from build123d import *

# Parameters (mm, degrees)
CROQUIS3_W              = 38
CROQUIS3_H              = 21.5
SALIENTE_EXTRUIR2_DEPTH = 60
CROQUIS4_R              = 4.1
CORTAR_EXTRUIR2_DEPTH   = 60
CROQUIS5_W              = 20
CROQUIS5_H              = 2
CORTAR_EXTRUIR4_DEPTH   = 39
CROQUIS6_R              = 3.5
CORTAR_EXTRUIR5_DEPTH   = 3
CROQUIS7_R              = 1.55
CORTAR_EXTRUIR6_DEPTH   = 22
CROQUIS8_R              = 4.5
CORTAR_EXTRUIR7_DEPTH   = 3
CROQUIS9_R              = 1.5
CORTAR_EXTRUIR8_DEPTH   = 15
CROQUIS10_W             = 38
CROQUIS10_H             = 0.5
CORTAR_EXTRUIR9_DEPTH   = 60


with BuildPart() as part:
    # Croquis3 → Saliente-Extruir2 (new body)
    with BuildSketch(Plane(origin=(0, 0, 0), x_dir=(0, 0, -1), z_dir=(1, 0, 0))):
        Rectangle(CROQUIS3_W, CROQUIS3_H)
    extrude(amount=SALIENTE_EXTRUIR2_DEPTH)

    # Croquis4 → Cortar-Extruir2 (cut)
    with BuildSketch(Plane(origin=(60, 0, 0), x_dir=(0, 0, -1), z_dir=(1, 0, 0))):
        with Locations((-10, 0)):
            Circle(CROQUIS4_R)
        with Locations((10, 0)):
            Circle(CROQUIS4_R)
    extrude(amount=-CORTAR_EXTRUIR2_DEPTH, mode=Mode.SUBTRACT)

    # Croquis5 → Cortar-Extruir4 (cut)
    with BuildSketch(Plane.XY.offset(19)):
        with Locations((50, 0)):
            Rectangle(CROQUIS5_W, CROQUIS5_H)
    extrude(amount=-CORTAR_EXTRUIR4_DEPTH, mode=Mode.SUBTRACT)

    # Croquis6 → Cortar-Extruir5 (cut)
    with BuildSketch(Plane.XZ.offset(10.75)):
        with Locations(Location((54, 0, 0), (0, 0, 270))):
            Circle(CROQUIS6_R)
    extrude(amount=-CORTAR_EXTRUIR5_DEPTH, mode=Mode.SUBTRACT)

    # Croquis7 → Cortar-Extruir6 (cut)
    with BuildSketch(Plane.XZ.offset(10.75)):
        with Locations(Location((54, 0, 0), (0, 0, 270))):
            Circle(CROQUIS7_R)
    extrude(amount=-CORTAR_EXTRUIR6_DEPTH, mode=Mode.SUBTRACT)

    # Croquis8 → Cortar-Extruir7 (cut)
    with BuildSketch(Plane(origin=(0, 10.75, 0), x_dir=(1, 0, 0), z_dir=(0, 1, 0))):
        with Locations(Location((54, 0, 0), (0, 0, 270))):
            Circle(CROQUIS8_R)
    extrude(amount=-CORTAR_EXTRUIR7_DEPTH, mode=Mode.SUBTRACT)

    # Croquis9 → Cortar-Extruir8 (cut)
    with BuildSketch(Plane(origin=(0, 10.75, 0), x_dir=(1, 0, 0), z_dir=(0, 1, 0))):
        with Locations(Location((30, 0, 0), (0, 0, 270))):
            Circle(CROQUIS9_R)
        with Locations(Location((15, 0, 0), (0, 0, 270))):
            Circle(CROQUIS9_R)
    extrude(amount=-CORTAR_EXTRUIR8_DEPTH, mode=Mode.SUBTRACT)

    # Croquis10 → Cortar-Extruir9 (cut)
    with BuildSketch(Plane.ZY):
        with Locations((0, 10.5)):
            Rectangle(CROQUIS10_W, CROQUIS10_H)
        with Locations((0, -10.5)):
            Rectangle(CROQUIS10_W, CROQUIS10_H)
    extrude(amount=-CORTAR_EXTRUIR9_DEPTH, mode=Mode.SUBTRACT)


solid = part.part
Work out the finished part from the listing and answer in its coordinate system (mm). A direction names the side the tool comes from. Coordinates: 2 decimals unless noted, no trailing zeros. Loops run counter-clockwise (first coordinate to the right, second up) from the corner with the lowest first, then second, coordinate; pieces in that order, holes last. Notation, with made-up numbers: M 61.5,-39 L 92.5,-39 A23 ccw 92.5,-21 Z; hole C 8.25,14.25 d10. An arc over 180 degrees is marked long. Answer in a Markdown table with one row per item. Add a question column.
1. Find section B-B, the plane x = 30. Write down the section's boundary in (y, z).
2. Find section C-C, the plane z = 10. Write down the section's boundary in (x, y).
3. Find section A-A, the plane y = 0. Write down the section's boundary in (x, z), then the cut area to 3 significant figures.
4. A tool of negligible diameter and unlimited length cuts with its end or side. For faces 1 (the cylindrical face through (31.265, 3.101, 0.806)), 2 (the flat face through (40, 0, -16)), 3 (the cylindrical face through (30.42, 1.23, -13.91)), 4 (the cylindrical face through (57.47, -9.02, 0.46)), 5 (the flat face through (30, 0, -19)), from which of +Z, -Z, +X, -X, +Y, -Y can it reach the whole face along a straight path? Write none if from no direction.
5. Consider L1, parallel to Z at x = 27.5, y = 0; L2, parallel to X at y = -0.75, z = 0; L3, parallel to Z at x = 49, y = -3. Determine where each line is inside the solid, lowest interval first.
6. The mould has two halves that part along X. Classify faces 6 (the cylindrical face through (55.537, 4.328, 0.202)), 7 (the flat face through (50, 1, 17)), 8 (the flat face through (40, 0, 0)): pulls with the +X half, pulls with the -X half, needs draft (parallel to the pull), parting line crosses it, or undercut.
7. Flat-ended cylindrical pins translate along their axes: P1, Ø10.5, axis at y = 0, z = -10, coming from the +X side; P2, Ø1, axis at y = 2.5, z = 9, coming from the -X side; P3, Ø2.5, axis at x = 52.5, z = -1, coming from the +Y side; P4, Ø5, axis at x = 54, z = 0, coming from the -Y side. Find the tip coordinate at first contact, or state that the pin passes through.
8. Find section D-D, the plane x = 11.5. Write down the section's boundary in (y, z).
Reported:
| question | item | result |
|---|---|---|
| 1 | outline | M -10.25,-19 L 10.25,-19 L 10.25,-1.5 L -4.25,-1.5 L -4.25,1.5 L 10.25,1.5 L 10.25,19 L -10.25,19 Z; hole C 0,-10 d8.2; hole C 0,10 d8.2 |
| 2 | outline | M 0,-10.25 L 60,-10.25 L 60,-4.1 L 0,-4.1 Z; M 0,4.1 L 60,4.1 L 60,10.25 L 0,10.25 Z |
| 3 | outline | M 0,-19 L 40,-19 L 40,-14.1 L 0,-14.1 Z; M 0,-5.9 L 40,-5.9 L 40,5.9 L 0,5.9 Z; M 0,14.1 L 40,14.1 L 40,19 L 0,19 Z; hole C 15,0 d3; hole C 30,0 d3 |
| 3 | area | 850 mm^2 |
| 4 | face 1 | +Y |
| 4 | face 2 | +Z, -Z, +X |
| 4 | face 3 | +X, -X |
| 4 | face 4 | -Y |
| 4 | face 5 | -Z, +X, -X, +Y, -Y |
| 5 | L1 | z = -19 to -14.1, -5.9 to 5.9, 14.1 to 19 |
| 5 | L2 | x = 0 to 13.5, 16.5 to 28.5, 31.5 to 40 |
| 5 | L3 | z = -19 to -12.79, -7.21 to 7.21, 12.79 to 19 |
| 6 | face 6 | undercut |
| 6 | face 7 | needs draft |
| 6 | face 8 | pulls with the +X half |
| 7 | P1 | stops at x = 60 |
| 7 | P2 | passes through |
| 7 | P3 | stops at y = 7.75 |
| 7 | P4 | stops at y = -7.75 |
| 8 | outline | M -10.25,-19 L 10.25,-19 L 10.25,19 L -10.25,19 Z; hole C 0,-10 d8.2; hole C 0,10 d8.2 |
